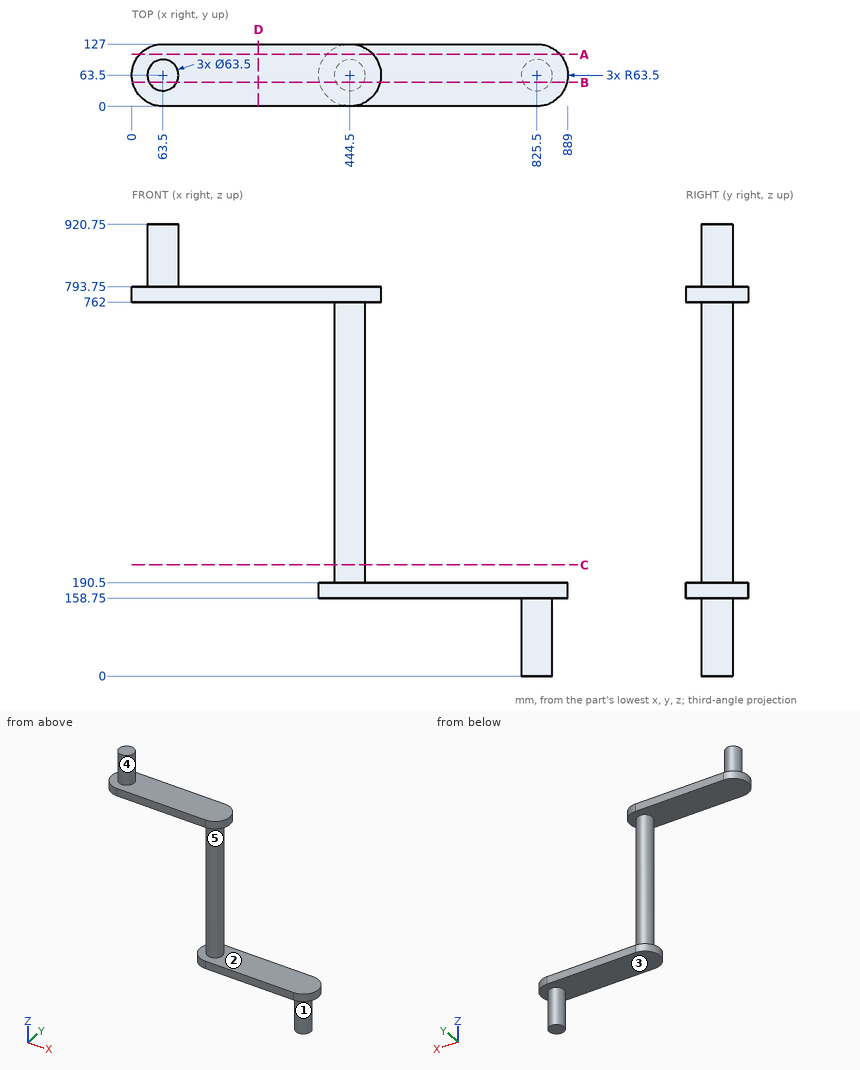
For this review, use the dimensioned drawing (mm, ordinates from the lowest corner) and the shaded views. A direction names the side the tool comes from. Round coordinates to 2 decimals unless told otherwise and drop trailing zeros. Write each loop counter-clockwise with the first axis right and the second up, starting at its lowest first coordinate (ties: lowest second). Pieces come first, ordered by that corner, then holes. Notation, with made-up numbers: (9.5, 24) - (14.5, 24) arc R22 cw to (14.5, 31) - close; hole circle Ø8 at (-25, 46.25). An arc over 180 degrees is marked (long way). One line per item, written item: value. Start each with the question number.
1. Consider section A-A on y = 106. Write out the cut boundary in (x, z).
2. To check wall thickness, follow L1, parallel to Z at x = 425.5, y = 8; L2, parallel to Z at x = 749, y = 116.5; L3, parallel to Z at x = 100, y = 46.5. State the ranges of each line that lie inside material, in increasing order. Write a range as from..to.
3. Consider section C-C on z = 226.5. Write out the cut boundary in (x, y), and give its area (3 significant figures).
4. Consider section D-D on x = 258. Write out the cut boundary in (y, z).
5. Machinability: for the marked faces 4 and 5, which of the approach directions +Z, -Z, +X, -X, +Y, -Y give a long, thin tool a straight path to every point of the face, cutting with its end or side? Answer none if there is none.
6. Consider section B-B on y = 49. Write out the cut boundary in (x, z), and give its area (3 significant figures).
7. The part is to be moulded in two halves that separate along Z. For the marked faces 1, 2 and 3, say which applies: released by +Z, released by -Z, zero draft, split by the parting line, or undercut.
8. Clearance check with flat-ended pins moving along their axes: P1, Ø3, axis at x = 309, y = 32.5, coming from the +Z side; P2, Ø3, axis at x = 775.5, y = 34, coming from the -Z side; P3, Ø1.5, axis at y = 75, z = 127, coming from the +X side. State where each tip first meets the part, or that it passes through.
Checks:
1. outline: (16.32, 762) - (491.68, 762) - (491.68, 793.75) - (16.32, 793.75) - close; (397.32, 158.75) - (872.68, 158.75) - (872.68, 190.5) - (397.32, 190.5) - close
2. L1: z = 158.75..190.5, 762..793.75
2. L2: z = 158.75..190.5
2. L3: z = 762..793.75
3. outline: circle Ø63.5 at (444.5, 63.5)
3. area: 3,170 mm^2
4. outline: (0, 762) - (127, 762) - (127, 793.75) - (0, 793.75) - close
5. face 4: +Z
5. face 5: none
6. outline: (1.68, 762) - (416.25, 762) - (416.25, 190.5) - (382.68, 190.5) - (382.68, 158.75) - (797.25, 158.75) - (797.25, 0) - (853.75, 0) - (853.75, 158.75) - (887.32, 158.75) - (887.32, 190.5) - (472.75, 190.5) - (472.75, 762) - (506.32, 762) - (506.32, 793.75) - (91.75, 793.75) - (91.75, 920.75) - (35.25, 920.75) - (35.25, 793.75) - (1.68, 793.75) - close
6. area: 80,500 mm^2
7. face 1: zero draft
7. face 2: undercut
7. face 3: released by -Z
8. P1: stops at z = 793.75
8. P2: stops at z = 158.75
8. P3: stops at x = 855.37
